Could you check a few things on this model? Use its own coordinates, in mm. A direction names the side the tool comes from. Round coordinates to 2 decimals unless told otherwise and drop trailing zeros. Write each loop counter-clockwise with the first axis right and the second up, starting at its lowest first coordinate (ties: lowest second). Pieces come first, ordered by that corner, then holes. Notation, with made-up numbers: (66, 31.25) -> (100, 31.25) arc R23 cw to (100, 54.25) -> close; hole circle Ø5 at (-4, 52.5). An arc over 180 degrees is marked (long way). One line per question, with ' | ' between items. Start each with the question number.
1. If I drill on line 1 along Y through (x, z) = (69, 16.5); line 2 along Z through (x, y) = (78.5, -9.5); line 3 along Z through (x, y) = (2, 0.5), over which ranges is the centre line in solid material (lowest first)? Write a range as [from, to].
2. Imagine slicing it at D-D, the plane z = 50. List the corners of the cut face in (x, y) for me, and give its area (3 significant figures).
3. Imagine slicing it at C-C, the plane y = 70.5. List the corners of the cut face in (x, z) for me, and give its area (3 significant figures).
4. Imagine slicing it at A-A, the plane x = 23. List the corners of the cut face in (y, z) for me, and give its area (3 significant figures).
5. Imagine slicing it at B-B, the plane x = 56. List the corners of the cut face in (y, z) for me.
6. For faces 1 (the flat face through (42, -7.493, 44)), 2 (the flat face through (42, 7.493, 44)), 3 (the flat face through (-6.79, 85.76, 12.52)), which set-ups out of +Z, -Z, +X, -X, +Y, -Y let a thin tool reach every point of the face, with its end or its side?
7. For pin 1 Ø14 at (x, z) = (76, 44.5) entering from -Y; pin 2 Ø4 at (x, y) = (3, -1.5) entering from +Z; pin 3 Ø8 at (x, y) = (36, 8.5) entering from +Z, each with a flat end and sliding along its axis, tell me the tip position at first contact or that it passes through.
from build123d import *

# Parameters (mm, degrees)
F0_R     = 42.8562327702
F1_DEPTH = 25.4
F2_DEPTH = 81.026
F3_R     = 33.2230738651
F4_R     = 5.5188922036
F5_R     = 5.08
F6_R     = 25.7152601394
F7_DEPTH = 59.182
F9_DEPTH = 7.493


with BuildPart() as f1:
    # F0 (on Top) → F1 (new body)
    with BuildSketch(Plane.XY):
        with BuildLine():
            ThreePointArc((-79.4371213769, -57.9695416598), (-28.2685910836, -47.036260575), (-5.3481783741, 0))
            ThreePointArc((-5.3481783741, 0), (-31.0855992866, 49.1102951098), (-86.1149848851, 55.8928198351))
            ThreePointArc((-86.1149848851, 55.8928198351), (-124.6918824332, -3.4966639305), (-79.4371213769, -57.9695416598))
        make_face()
        with Locations((-65.0712549686, 0)):
            Circle(F0_R, mode=Mode.SUBTRACT)
        with BuildLine():
            ThreePointArc((-86.1149848851, 55.8928198351), (-31.0855992866, 49.1102951098), (-5.3481783741, 0))
            ThreePointArc((-5.3481783741, 0), (-28.2685910836, -47.036260575), (-79.4371213769, -57.9695416598))
            Line((-79.4371213769, -57.9695416598), (120.1632661658, -107.4340090401))
            Line((120.1632661658, -107.4340090401), (114.0664431846, 131.2614256598))
            Line((114.0664431846, 131.2614256598), (-86.1149848851, 55.8928198351))
        make_face()
    extrude(amount=F1_DEPTH)

    # F0 (on Top) → F2 (join)
    with BuildSketch(Plane.XY):
        with BuildLine():
            ThreePointArc((-79.4371213769, -57.9695416598), (-28.2685910836, -47.036260575), (-5.3481783741, 0))
            ThreePointArc((-5.3481783741, 0), (-31.0855992866, 49.1102951098), (-86.1149848851, 55.8928198351))
            ThreePointArc((-86.1149848851, 55.8928198351), (-124.6918824332, -3.4966639305), (-79.4371213769, -57.9695416598))
        make_face()
        with Locations((-65.0712549686, 0)):
            Circle(F0_R, mode=Mode.SUBTRACT)
    extrude(amount=F2_DEPTH)

    # F3
    f3_edges = [f1.edges().sort_by_distance(p)[0] for p in [
        (120.163266, -107.434009, 12.7),
        (114.066443, 131.261426, 12.7),
    ]]
    fillet(f3_edges, radius=F3_R)

    # F4
    f4_edges = [f1.edges().sort_by_distance(p)[0] for p in [
        (-107.927488, 0, 81.026),
    ]]
    fillet(f4_edges, radius=F4_R)

    # F5
    f5_edges = [f1.edges().sort_by_distance(p)[0] for p in [
        (-44.027525, -55.89282, 81.026),
    ]]
    fillet(f5_edges, radius=F5_R)

    # F6 (on Top) → F7 (cut)
    with BuildSketch(Plane.XY):
        with Locations((72.004429996, -49.6582314372)):
            Circle(F6_R)
        with Locations((69.8762312531, 53.9146512747)):
            Circle(F6_R)
    extrude(amount=F7_DEPTH, mode=Mode.SUBTRACT)

    # F8 (on Front) → F9 (join, symmetric)
    with BuildSketch(Plane.XZ):
        Polygon((-11.3121019676, 25.740753975), (118.4722334146, 26.3785142452), (-11.3121019676, 74.8483398067), align=None)
    extrude(amount=F9_DEPTH, both=True)


solid = f1.part
Geometry results:
1) line 1: y = [-94.75, -75.2], [-24.12, 28.21], [79.61, 114.29] | line 2: z = [0, 25.4] | line 3: z = [0, 25.4], [25.81, 69.88]
2) outline: (-5.82, -7.49) -> (55.22, -7.49) -> (55.22, 7.49) -> (-5.82, 7.49) arc R59.72 ccw (long way) to start; hole circle Ø85.71 at (-65.07, 0) | area: 6,350 mm2
3) outline: (-47.32, 0) -> (50.22, 0) -> (50.22, 25.4) -> (-47.32, 25.4) -> close; (89.53, 0) -> (115.62, 0) -> (115.62, 25.4) -> (89.53, 25.4) -> close | area: 3,140 mm2
4) outline: (-83.36, 0) -> (96.97, 0) -> (96.97, 25.4) -> (-83.36, 25.4) -> close; (-7.49, 25.91) -> (7.49, 25.91) -> (7.49, 62.03) -> (-7.49, 62.03) -> close | area: 5,120 mm2
5) outline: (-91.53, 0) -> (-69.79, 0) -> (-69.79, 25.4) -> (-91.53, 25.4) -> close; (-29.53, 0) -> (32.26, 0) -> (32.26, 25.4) -> (-29.53, 25.4) -> close; (-7.49, 26.07) -> (7.49, 26.07) -> (7.49, 49.71) -> (-7.49, 49.71) -> close; (75.56, 0) -> (109.4, 0) -> (109.4, 25.4) -> (75.56, 25.4) -> close
6) face 1: +Z, +X, -Y | face 2: +Z, +X, +Y | face 3: +Z, -Z, -X, +Y
7) pin 1: stops at y = -7.49 | pin 2: stops at z = 70.25 | pin 3: stops at z = 58.62
